The model under review builds one solid part; all positions refer to its coordinate system, in mm. A direction names the side the tool comes from. Round coordinates to 2 decimals unless told otherwise and drop trailing zeros. Order: outer loops, then holes, each group sorted by start corner. A loop starts at its lowest first (then second) coordinate and runs counter-clockwise, first axis right, second up. Notation, with made-up numbers: M 73,-6 L 130,-6 A17 ccw 130,25 Z; hole C 32,77 d5. An arc over 180 degrees is marked long. Answer as a JSON object with one key per item and string values. Group by question number.
1. Machinability: for faces 4 (the face through (-17, 6, -17)), 5 (the face through (-19.524, 4.056, -4.336)), which of the approach directions +Z, -Z, +X, -X, +Y, -Y give a long, thin tool a straight path to every point of the face, cutting with its end or side? Answer none if there is none.
2. Add section A-A on x = 0. State the section outline as (y, z) points, and give its area (3 significant figures).
3. Add section D-D on y = 7.25. State the section outline as (x, z) points.
4. Add section B-B on z = 0. State the section outline as (x, y) points.
5. Mouldability with a two-part tool opening along Z and no side actions: class faces 1 (the face through (7.509, 2.958, 23.846)), 2 (the face through (14.531, 6.028, -15.846)), 3 (the face through (-13, 8, 16)) as released by +Z, released by -Z, zero draft, split by the parting line, or undercut.
6. Clearance check with flat-ended pins moving along their axes: P1, Ø2, axis at x = 11, y = 1.5, coming from the +Z side; P2, Ø4, axis at y = 3, z = 5, coming from the -X side; P3, Ø4, axis at y = 3.5, z = -12.5, coming from the +X side. State where each tip first meets the part, or that it passes through.
7. To check wall thickness, follow probe 1 along X at (y, z) = (5, 0); probe 2 along X at (y, z) = (2.75, 0); probe 3 along X at (y, z) = (5.25, -11.5). State the ranges of each line that lie inside material, in increasing order. Write a range as [from, to].
8. Add section C-C on y = 0.75. State the section outline as (x, z) points, and give its area (3 significant figures).
```python
from build123d import *

# Parameters (mm, degrees)
SKETCH1_R           = 25
BOSS_EXTRUDE1_DEPTH = 8
SKETCH2_R           = 23.5
SKETCH2_R_2         = 21.5
CUT_EXTRUDE1_DEPTH  = 4
SKETCH3_R           = 25
SKETCH3_R_2         = 23.5
CUT_EXTRUDE2_DEPTH  = 2
CUT_EXTRUDE3_REACH  = 38.249
SKETCH4_R           = 20


with BuildPart() as part:
    # Sketch1 → Boss-Extrude1 (new body)
    with BuildSketch(Plane(origin=(0, 0, 0), x_dir=(1, 0, 0), z_dir=(0, 1, 0))):
        with Locations(Location((0, 0, 0), (0, 0, 270))):
            Circle(SKETCH1_R)
    extrude(amount=BOSS_EXTRUDE1_DEPTH)

    # Sketch2 → Cut-Extrude1 (cut)
    with BuildSketch(Plane(origin=(0, 8, 0), x_dir=(1, 0, 0), z_dir=(0, 1, 0))):
        with Locations(Location((0, 0, 0), (0, 0, 270))):
            Circle(SKETCH2_R)
        with Locations(Location((0, 0, 0), (0, 0, 270))):
            Circle(SKETCH2_R_2, mode=Mode.SUBTRACT)
    extrude(amount=-CUT_EXTRUDE1_DEPTH, mode=Mode.SUBTRACT)

    # Sketch3 → Cut-Extrude2 (cut)
    with BuildSketch(Plane(origin=(0, 8, 0), x_dir=(1, 0, 0), z_dir=(0, 1, 0))):
        with Locations(Location((0, 0, 0), (0, 0, 270))):
            Circle(SKETCH3_R)
        with Locations(Location((0, 0, 0), (0, 0, 270))):
            Circle(SKETCH3_R_2, mode=Mode.SUBTRACT)
    extrude(amount=-CUT_EXTRUDE2_DEPTH, mode=Mode.SUBTRACT)

    # Sketch4 → Cut-Extrude3 (cut, up to next)
    with BuildSketch(Plane(origin=(0, 8, 0), x_dir=(1, 0, 0), z_dir=(0, 1, 0)), mode=Mode.PRIVATE) as cut_extrude3_sk1:
        with Locations(Location((0, 0, 0), (0, 0, 270))):
            Circle(SKETCH4_R)
    cut_extrude3_tool1 = extrude(cut_extrude3_sk1.sketch, amount=-CUT_EXTRUDE3_REACH, mode=Mode.PRIVATE) & part.part
    add(cut_extrude3_tool1.solids().sort_by_distance((0, 8, 0))[0], mode=Mode.SUBTRACT)


solid = part.part
```
Recorded:
{
 "1": {"face 4": "+Y", "face 5": "+Y, -Y"},
 "2": {"outline": "M 0,-25 L 6,-25 L 6,-23.5 L 4,-23.5 L 4,-21.5 L 8,-21.5 L 8,-20 L 0,-20 Z; M 0,20 L 8,20 L 8,21.5 L 4,21.5 L 4,23.5 L 6,23.5 L 6,25 L 0,25 Z", "area": "58.0 mm²"},
 "3": {"outline": "C 0,0 d43; hole C 0,0 d40"},
 "4": {"outline": "M -25,0 L -20,0 L -20,8 L -21.5,8 L -21.5,4 L -23.5,4 L -23.5,6 L -25,6 Z; M 20,0 L 25,0 L 25,6 L 23.5,6 L 23.5,4 L 21.5,4 L 21.5,8 L 20,8 Z"},
 "5": {"face 1": "split by the parting line", "face 2": "undercut", "face 3": "zero draft"},
 "6": {"P1": "stops at z = 22.91", "P2": "stops at x = -24.82", "P3": "stops at x = 22.69"},
 "7": {"probe 1": "x = [-25, -23.5], [-21.5, -20], [20, 21.5], [23.5, 25]", "probe 2": "x = [-25, -20], [20, 25]", "probe 3": "x = [-22.2, -20.49], [-18.17, -16.36], [16.36, 18.17], [20.49, 22.2]"},
 "8": {"outline": "C 0,0 d50; hole C 0,0 d40", "area": "707 mm²"}
}
